```python
from build123d import *

# Parameters (mm, degrees)
SKETCH1_W           = 17.4
SKETCH1_H           = 15.2
SKETCH1_R           = 1.65
BOSS_EXTRUDE1_DEPTH = 5
SKETCH2_W           = 17.4
SKETCH2_H           = 15.2
SKETCH2_W_2         = 15.4
SKETCH2_H_2         = 13.2
BOSS_EXTRUDE2_DEPTH = 1.2
CUT_EXTRUDE1_START  = -1
SKETCH3_R           = 3.1
CUT_EXTRUDE1_DEPTH  = 2.2
SKETCH4_R           = 2.25
CUT_EXTRUDE2_DEPTH  = 1
SKETCH6_W           = 4.5
SKETCH6_H           = 4.5
CUT_EXTRUDE4_DEPTH  = 0.12
SKETCH7_W           = 17.4
SKETCH7_H           = 15.2
SKETCH7_R           = 4.23
BOSS_EXTRUDE3_DEPTH = 10
CHAMFER1_SIZE       = 3
CHAMFER1_SIZE2      = 0.528980942
SKETCH9_R           = 1.85
BOSS_EXTRUDE5_DEPTH = 10
CUT_EXTRUDE5_DEPTH  = 16.2
CHAMFER3_SIZE       = 1.4
CHAMFER3_SIZE2      = 2.424871131


with BuildPart() as part:
    # Sketch1 → Boss-Extrude1 (new body)
    with BuildSketch(Plane.XY):
        Rectangle(SKETCH1_W, SKETCH1_H)
        Circle(SKETCH1_R, mode=Mode.SUBTRACT)
    extrude(amount=BOSS_EXTRUDE1_DEPTH)

    # Sketch2 → Boss-Extrude2 (add)
    with BuildSketch(Plane.XY.offset(5)):
        Rectangle(SKETCH2_W, SKETCH2_H)
        Rectangle(SKETCH2_W_2, SKETCH2_H_2, mode=Mode.SUBTRACT)
    extrude(amount=BOSS_EXTRUDE2_DEPTH)

    # Sketch3 → Cut-Extrude1 (cut)
    with BuildSketch(Plane.XY.offset(5).offset(CUT_EXTRUDE1_START)):
        Circle(SKETCH3_R)
    extrude(amount=-CUT_EXTRUDE1_DEPTH, mode=Mode.SUBTRACT)

    # Sketch4 → Cut-Extrude2 (cut)
    with BuildSketch(Plane.XY.offset(5)):
        Circle(SKETCH4_R)
    extrude(amount=-CUT_EXTRUDE2_DEPTH, mode=Mode.SUBTRACT)

    # Sketch6 → Cut-Extrude4 (cut)
    with BuildSketch(Plane(origin=(0, 0, 4), x_dir=(-1, 0, 0), z_dir=(0, 0, -1))):
        Rectangle(SKETCH6_W, SKETCH6_H)
    extrude(amount=-CUT_EXTRUDE4_DEPTH, mode=Mode.SUBTRACT)

    # Sketch7 → Boss-Extrude3 (add)
    with BuildSketch(Plane(origin=(0, 0, 0), x_dir=(-1, 0, 0), z_dir=(0, 0, -1))):
        Rectangle(SKETCH7_W, SKETCH7_H)
        Circle(SKETCH7_R, mode=Mode.SUBTRACT)
    extrude(amount=BOSS_EXTRUDE3_DEPTH)

    # Chamfer1
    chamfer1_edges = [part.edges().sort_by_distance(p)[0] for p in [
        (4.23, 0, -10),
    ]]
    chamfer1_side = [part.faces().sort_by_distance(p)[0] for p in [
        (4.23, 0, -5),
    ]]
    chamfer(chamfer1_edges, length=CHAMFER1_SIZE, length2=CHAMFER1_SIZE2, reference=chamfer1_side[0])

    # Sketch9 → Boss-Extrude5 (add)
    with BuildSketch(Plane.XY.offset(6.2)):
        with BuildLine():
            Line((8.7, 7.6), (8.7, -7.6))
            Line((8.7, -7.6), (11.756854249, -7.6))
            Line((11.756854249, -7.6), (16.528427125, -2.828427125))
            ThreePointArc((16.528427125, -2.828427125), (17.7, 0), (16.528427125, 2.828427125))
            Line((16.528427125, 2.828427125), (11.756854249, 7.6))
            Line((11.756854249, 7.6), (8.7, 7.6))
        make_face()
        with Locations((13.7, 0)):
            Circle(SKETCH9_R, mode=Mode.SUBTRACT)
        with BuildLine():
            Line((-8.7, 7.6), (-8.7, -7.6))
            Line((-8.7, -7.6), (-11.756854249, -7.6))
            Line((-11.756854249, -7.6), (-16.528427125, -2.828427125))
            ThreePointArc((-16.528427125, -2.828427125), (-17.7, 0), (-16.528427125, 2.828427125))
            Line((-16.528427125, 2.828427125), (-11.756854249, 7.6))
            Line((-11.756854249, 7.6), (-8.7, 7.6))
        make_face()
        with Locations((-13.7, 0)):
            Circle(SKETCH9_R, mode=Mode.SUBTRACT)
    extrude(amount=-BOSS_EXTRUDE5_DEPTH)

    # Sketch10 → Cut-Extrude5 (cut, through all)
    with BuildSketch(Plane.XZ.offset(7.6)):
        Polygon((-8.7, -3.8), (-19.607158184, 3.837274381), (-19.607158184, -3.8), align=None)
        Polygon((19.607158184, -3.8), (8.7, -3.8), (19.607158184, 3.837274381), align=None)
    extrude(amount=-CUT_EXTRUDE5_DEPTH, mode=Mode.SUBTRACT)

    # Chamfer3
    chamfer3_edges = [part.edges().sort_by_distance(p)[0] for p in [
        (4.23, 0, 0),
    ]]
    chamfer3_side = [part.faces().sort_by_distance(p)[0] for p in [
        (4.23, 0, -3.5),
    ]]
    chamfer(chamfer3_edges, length=CHAMFER3_SIZE, length2=CHAMFER3_SIZE2, reference=chamfer3_side[0])


solid = part.part
```
Here's how the part is built. I have some questions about the finished solid (model axes, mm). A direction names the side the tool comes from. Give positions to 0.01 mm unless a question says otherwise; leave off trailing zeros. Loops run counter-clockwise (first coordinate to the right, second up) from the corner with the lowest first, then second, coordinate; pieces in that order, holes last. Notation, with made-up numbers: M 60,45 L 78,45 A21 cw 78,76 Z; hole C 10,62.5 d8. An arc over 180 degrees is marked long. Use one line per item in the form item = value. Start each with the question number.
Q1. If we section it at C-C (y = 1): State how many separate pieces and enclosed holes the cut face has, then the cut area to 3 significant figures.
Q2. If we section it at A-A (x = -14): Write out the boundary of the cut face in (y, z).
Q3. Thinking about a two-plate mould opening in Z: for faces 6 (the flat face through (11.14, -0.11, -2.09)), 7 (the flat face through (-2, 2, 4.12)), 8 (the flat face through (0, 6.6, 6)), which applies, +Z half, -Z half, draft (parallel to the pull), parting line (faces both ways), or undercut?
Q4. I need wall thicknesses on line 1 along X through (y, z) = (0, 3); line 2 along Y through (x, z) = (0, -3.6); line 3 along Y through (x, z) = (0, 3.5). Which ranges of each line are inside material? Lowest first, please.
Q5. Will these pins go through, and if not, where does the flat tip stop? pin 1 Ø4 at (y, z) = (-5.5, 2) entering from +X; pin 2 Ø0.6 at (y, z) = (1.5, 5.5) entering from +X; pin 3 Ø0.9 at (x, y) = (0.5, 2.5) entering from -Z.
Q6. If we section it at B-B (x = 15): Write out the boundary of the cut face in (y, z).
Q7. Which directions (+Z, -Z, +X, -X, +Y, -Y) give clear straight access to the entire face, cutting with the end or side of a thin tool? Please do faces 1 (the flat face through (8.7, 0, -7)), 2 (the flat face through (0, -6.6, 6)), 3 (the flat face through (-8.7, 0, -7)), 4 (the cylindrical face through (11.85, 0.08, 3.18)), 5 (the flat face through (2.6, 0, 4)).
Taken from the geometry:
q1.separate_pieces = 4
q1.enclosed_holes = 0
q1.area = 243 mm^2
q2.outline = M -5.36,-0.09 L -1.83,-0.09 L -1.83,6.2 L -5.36,6.2 Z; M 1.83,-0.09 L 5.36,-0.09 L 5.36,6.2 L 1.83,6.2 Z
q3.face_6 = -Z half
q3.face_7 = undercut
q3.face_8 = draft
q4.line_1 = -17.7 to -15.55, -11.85 to -3.1, 3.1 to 11.85, 15.55 to 17.7
q4.line_2 = -7.6 to -4.23, 4.23 to 7.6
q4.line_3 = -7.6 to -3.1, 3.1 to 7.6
q5.pin_1 = 15.86
q5.pin_2 = 17.52
q5.pin_3 = -0.69
q6.outline = M -4.36,0.61 L -1.32,0.61 L -1.32,6.2 L -4.36,6.2 Z; M 1.32,0.61 L 4.36,0.61 L 4.36,6.2 L 1.32,6.2 Z
q7.face_1 = -Z, +X, +Y, -Y
q7.face_2 = +Z
q7.face_3 = -Z, -X, +Y, -Y
q7.face_4 = +Z, -Z
q7.face_5 = none
